from build123d import *

# Parameters (mm, degrees)
SKETCH1_R           = 95
BOSS_EXTRUDE1_DEPTH = 10
SKETCH2_R           = 65
BOSS_EXTRUDE2_DEPTH = 10
SKETCH3_R           = 57.5
CUT_EXTRUDE1_DEPTH  = 10
SKETCH4_R           = 7
CUT_EXTRUDE2_DEPTH  = 136.830777072
SKETCH5_R           = 30.75
CUT_EXTRUDE3_DEPTH  = 136.830777072


with BuildPart() as part:
    # Sketch1 → Boss-Extrude1 (new, symmetric)
    with BuildSketch(Plane(origin=(0, 0, 0), x_dir=(1, 0, 0), z_dir=(0, 1, 0))):
        with Locations(Location((0, 0, 0), (0, 0, 270))):
            Circle(SKETCH1_R)
    extrude(amount=BOSS_EXTRUDE1_DEPTH, both=True)

    # Sketch2 → Boss-Extrude2 (add)
    with BuildSketch(Plane(origin=(0, 10, 0), x_dir=(1, 0, 0), z_dir=(0, 1, 0))):
        with Locations(Location((0, 0, 0), (0, 0, 270))):
            Circle(SKETCH2_R)
    extrude(amount=BOSS_EXTRUDE2_DEPTH)

    # Sketch3 → Cut-Extrude1 (cut)
    with BuildSketch(Plane(origin=(0, 20, 0), x_dir=(1, 0, 0), z_dir=(0, 1, 0))):
        with Locations(Location((0, 0, 0), (0, 0, 270))):
            Circle(SKETCH3_R)
    extrude(amount=-CUT_EXTRUDE1_DEPTH, mode=Mode.SUBTRACT)

    # Sketch4 → Cut-Extrude2 (cut, through all)
    with BuildSketch(Plane(origin=(0, 10, 0), x_dir=(1, 0, 0), z_dir=(0, 1, 0))):
        with Locations(Location((0, 80, 0), (0, 0, 270))):
            Circle(SKETCH4_R)
        with Locations(Location((80, 0, 0), (0, 0, 270))):
            Circle(SKETCH4_R)
        with Locations(Location((0, -80, 0), (0, 0, 270))):
            Circle(SKETCH4_R)
        with Locations(Location((-80, 0, 0), (0, 0, 270))):
            Circle(SKETCH4_R)
    extrude(amount=-CUT_EXTRUDE2_DEPTH, mode=Mode.SUBTRACT)

    # Sketch5 → Cut-Extrude3 (cut, through all)
    with BuildSketch(Plane(origin=(0, 10, 0), x_dir=(1, 0, 0), z_dir=(0, 1, 0))):
        with Locations(Location((0, 0, 0), (0, 0, 270))):
            Circle(SKETCH5_R)
    extrude(amount=-CUT_EXTRUDE3_DEPTH, mode=Mode.SUBTRACT)

    # Sketch6 → Cut-Revolve3 (revolve, cut)
    with BuildSketch(Plane(origin=(0, 0, 0), x_dir=(0, 0, -1), z_dir=(1, 0, 0))):
        Polygon((0, 3.5), (-30.814786926, 3.5), (-38.5, 2.5), (-38.5, -2.5), (-30.814786926, -3.5), (0, -3.5), align=None)
    revolve(axis=Axis((0, 3.5, 0), (0, -1, 0)), mode=Mode.SUBTRACT)


solid = part.part
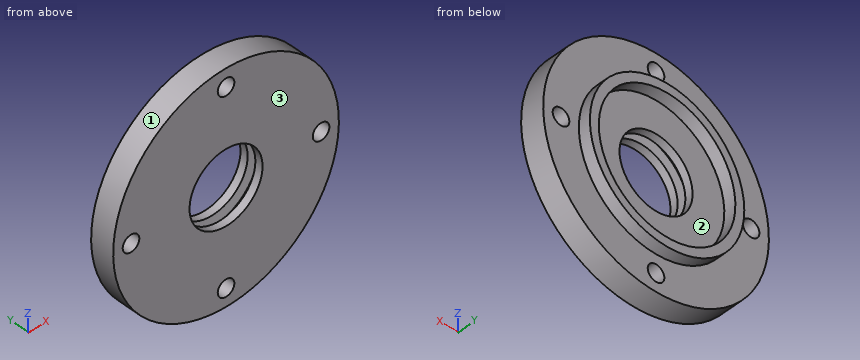
Can you work these out from the model? Positions are in its coordinate system, mm. Face numbers are marked on the shaded views. Round coordinates to 2 decimals unless told otherwise and drop trailing zeros. Loops run counter-clockwise (first coordinate to the right, second up) from the corner with the lowest first, then second, coordinate; pieces in that order, holes last. Notation, with made-up numbers: (9, 57.5) - (21, 57.5) arc R11 ccw to (21, 72.5) - close; hole circle Ø6 at (33.25, -26). An arc over 180 degrees is marked (long way). Write item = value, one per line. Start each with the question number.
(1) If we section it at B-B (z = -80): Please give me the cut outline in (x, y).
(2) If we mould it in two halves opening along Z, with no side actions, what happens to the marked faces 1, 2 and 3? For each: released by +Z, released by -Z, zero draft, split by the parting line, or undercut.
(3) If we section it at C-C (x = 0): Give the number of separate pieces and of enclosed holes in the cut face, and give its area (3 significant figures).
(4) If we section it at D-D (x = 80): Please give me the cut outline in (y, z).
(5) If we section it at A-A (y = 6.5): Please give me the cut outline in (x, z), and give its area (3 significant figures).
(6) If I drill on probe 1 along X at (y, z) = (-8, 0); probe 2 along X at (y, z) = (14.75, 0); probe 3 along Y at (x, z) = (-11, 67), over which ranges is the centre line in solid material (lowest first)? Write a range as [from, to].
(7) For P1, Ø4, axis at x = 19.5, y = 1.5, coming from the -Z side; P2, Ø12, axis at y = -2.5, z = -46.5, coming from the -X side; P3, Ø2, axis at x = 27.5, y = 16, coming from the +Z side, each with a flat end and sliding along its axis, tell me the tip position at first contact or that it passes through.
Ans:
q1.outline = (-51.23, -10) - (-7, -10) - (-7, 10) - (-51.23, 10) - close; (7, -10) - (51.23, -10) - (51.23, 10) - (7, 10) - close
q2.face_1 = split by the parting line
q2.face_2 = undercut
q2.face_3 = zero draft
q3.separate_pieces = 4
q3.enclosed_holes = 0
q3.area = 2,070 mm²
q4.outline = (-10, -51.23) - (10, -51.23) - (10, -7) - (-10, -7) - close; (-10, 7) - (10, 7) - (10, 51.23) - (-10, 51.23) - close
q5.outline = circle Ø190 at (0, 0); hole circle Ø14 at (-80, 0); hole circle Ø61.5 at (0, 0); hole circle Ø14 at (0, -80); hole circle Ø14 at (0, 80); hole circle Ø14 at (80, 0)
q5.area = 24,800 mm²
q6.probe_1 = [-95, -87], [-73, -30.75], [30.75, 73], [87, 95]
q6.probe_2 = [-65, -57.5], [57.5, 65]
q6.probe_3 = [-10, 10]
q7.P1 = -93.37
q7.P2 = -85.93
q7.P3 = 59.35
